Design review of the part built by this model. Coordinates are the model's own, in mm. Give positions to 0.01 mm unless a question says otherwise; leave off trailing zeros. Loops run counter-clockwise (first coordinate to the right, second up) from the corner with the lowest first, then second, coordinate; pieces in that order, holes last.
from build123d import *

# Parameters (mm, degrees)
F0_W        = 22.987
F0_H        = 25.4
F1_DEPTH    = 25.4
F3_D        = 6.8
F4_SIZE     = 6.35
F5_SIZE     = 6.35
F6_T1_DEPTH = 140.0532259942


# Not quite as in the source:
# - a fillet or chamfer that OpenCascade refuses, or shapes differently, is made with other operations: its cross-section is extruded or revolved along the edge and cut away or added


with BuildPart() as f1:
    # F0 (on Front) → F1 (new body, symmetric)
    with BuildSketch(Plane.XZ):
        Rectangle(F0_W, F0_H)
    extrude(amount=F1_DEPTH, both=True)

    # F3 (through all)
    with Locations(Plane.XY.offset(12.7)):
        with Locations((0, 0)):
            Hole(F3_D / 2)

    # F4
    f4_edges = [f1.edges().sort_by_distance(p)[0] for p in [
        (11.4935, -25.4, 0),
    ]]
    chamfer(f4_edges, length=F4_SIZE)

    # F5
    f5_edges = [f1.edges().sort_by_distance(p)[0] for p in [
        (11.4935, 25.4, 0),
    ]]
    chamfer(f5_edges, length=F5_SIZE)

    # F6: chamfer of 19.05 x 19.812 on 1 edges, made by hand

    # F6_s2 → F6_t1 (cut)
    with BuildSketch(Plane.XZ.offset(-70.0266129971)):
        Polygon((11.4935, 6.35), (-8.3185, -12.7), (11.4935, -12.7), align=None)
    extrude(amount=F6_T1_DEPTH, mode=Mode.SUBTRACT)


solid = f1.part
Q1. Take a section at C-C (y = 0). Give the boundary of the cut face in (x, z).
Results:
outline: (-11.49, -12.7) - (-8.32, -12.7) - (-3.4, -7.97) - (-3.4, 12.7) - (-11.49, 12.7) - close; (3.4, -1.43) - (11.49, 6.35) - (11.49, 12.7) - (3.4, 12.7) - close
Q2. Insertion check: pin 1 (9 mm diameter, centred on x = 0, y = 0, fed in from -Z); pin 2 (8 mm diameter, centred on x = 1, y = -9.5, fed in from -Z). Each pin has a flat end and moves straight along its axis. Give the tip position at first contact, or say it passes through.
Results:
pin 1: stops at z = -9.03
pin 2: stops at z = -7.59
Q3. Take a section at B-B (x = 0). Give the boundary of the cut face in (y, z).
Results:
outline: (-25.4, -4.7) - (-3.4, -4.7) - (-3.4, 12.7) - (-25.4, 12.7) - close; (3.4, -4.7) - (25.4, -4.7) - (25.4, 12.7) - (3.4, 12.7) - close
Q4. Draft analysis for pull direction X (two halves, no side actions). For faces 1 (the face through (11.494, 0, 9)), 2 (the face through (-3.14, -1.3, 4.52)), 3 (the face through (-10, 0, -12.7)), state which applies: pulls with the +X half, pulls with the -X half, needs draft (parallel to the pull), parting line crosses it, or undercut.
Results:
face 1: pulls with the +X half
face 2: undercut
face 3: needs draft
Q5. Take a section at D-D (y = 13). Give the boundary of the cut face in (x, z).
Results:
outline: (-11.49, -12.7) - (-8.32, -12.7) - (11.49, 6.35) - (11.49, 12.7) - (-11.49, 12.7) - close
Q6. Wall thickness on line 1 (Y direction, x = 0, z = -1.75); line 2 (X direction, y = 0, z = 8.75); line 3 (X direction, y = 0, z = -2.75): over which ranges is each line inside the solid? List them lowest first.
Results:
line 1: y = -25.4 to -3.4, 3.4 to 25.4
line 2: x = -11.49 to -3.4, 3.4 to 11.49
line 3: x = -11.49 to -3.4
Q7. Take a section at A-A (z = 10.75). Give the boundary of the cut face in (x, y).
Results:
outline: (-11.49, -25.4) - (5.14, -25.4) - (11.49, -19.05) - (11.49, 19.05) - (5.14, 25.4) - (-11.49, 25.4) - close; hole circle Ø6.8 at (0, 0)
